Source: three-view drawing plus pictorial views. Frame: mm from the lowest corner of the part. A direction names the side the tool comes from. Coordinates: 2 decimals unless noted, no trailing zeros. Order: outer loops, then holes, each group sorted by start corner. A loop starts at its lowest first (then second) coordinate and runs counter-clockwise, first axis right, second up. Notation, with made-up numbers: (54.5, 83) -> (102.5, 83) arc R12 ccw to (102.5, 103) -> close; hole circle Ø6 at (25, 60.25). An arc over 180 degrees is marked (long way). Use one line per item in the form item = value. Start each with the question number.
1) Ray query, line 1 along Z through (x, y) = (132.5, 16.5); line 2 along X through (y, z) = (7.5, 15); line 3 along Y through (x, z) = (85.5, 62.5). Return the intervals inside material, ascending.
2) Section query A-A on y = 21. Output: boundary loops of the cut face in (x, z).
3) Section query B-B on z = 40. Output: boundary loops of the cut face in (x, y), then the cut area to 3 significant figures.
4) Draft query along X for the marked faces 1, 2, 3 and 4. Return one class per face: pulls with the +X half, pulls with the -X half, needs draft (parallel to the pull), parting line crosses it, or undercut.
5) Pin query (flat end, axial travel): pin 1 (8 mm diameter, centred on x = 114, z = 23, fed in from +Y). Return the tip coordinate at first contact, or that it passes through.
6) Section query C-C on x = 145.5. Output: boundary loops of the cut face in (y, z).
7) Access query for the marked faces 5 and 6. Directions: +Z, -Z, +X, -X, +Y, -Y. A direction counts if a zero-diameter tool reaches every point of the face in a straight line with its end or side. Return the directions, or none.
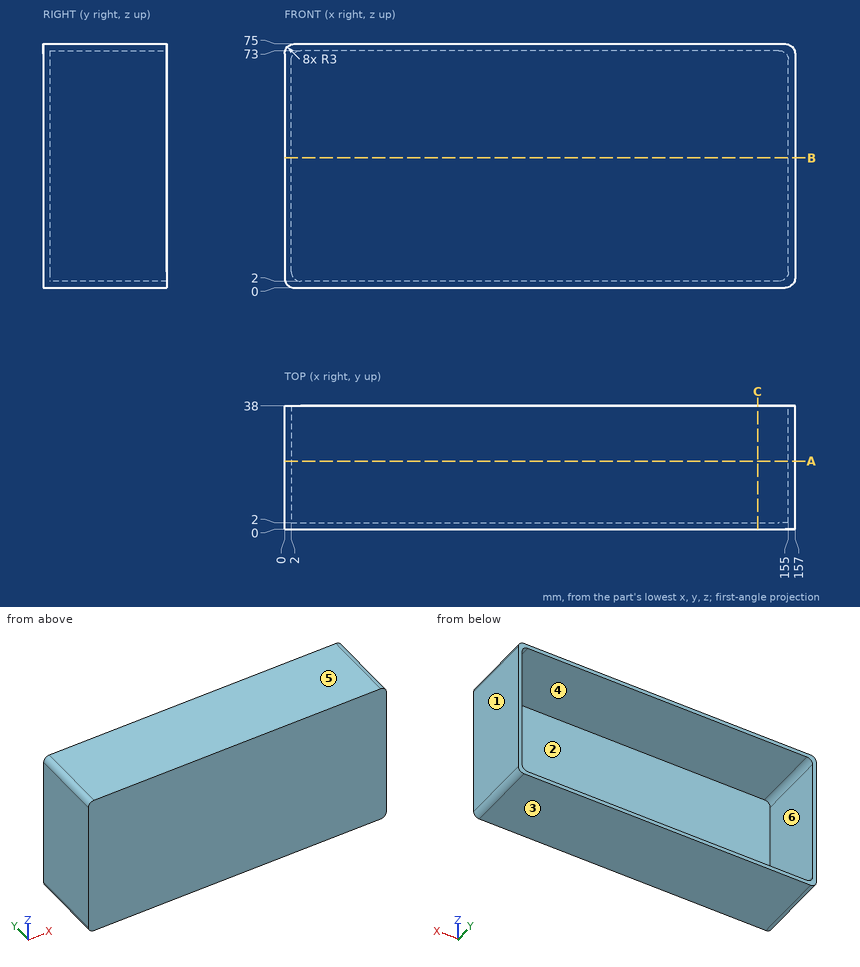
Answers below:
q1.line_1 = 0 to 2, 73 to 75
q1.line_2 = 0 to 2, 155 to 157
q1.line_3 = 0 to 2
q2.outline = (0, 3) arc R3 ccw to (3, 0) -> (154, 0) arc R3 ccw to (157, 3) -> (157, 72) arc R3 ccw to (154, 75) -> (3, 75) arc R3 ccw to (0, 72) -> close; hole (2, 5) arc R3 ccw to (5, 2) -> (152, 2) arc R3 ccw to (155, 5) -> (155, 70) arc R3 ccw to (152, 73) -> (5, 73) arc R3 ccw to (2, 70) -> close
q3.outline = (0, 0) -> (157, 0) -> (157, 38) -> (155, 38) -> (155, 2) -> (2, 2) -> (2, 38) -> (0, 38) -> close
q3.area = 458 mm^2
q4.face_1 = pulls with the +X half
q4.face_2 = undercut
q4.face_3 = needs draft
q4.face_4 = undercut
q5.pin_1 = 2
q6.outline = (0, 0) -> (38, 0) -> (38, 2) -> (2, 2) -> (2, 73) -> (38, 73) -> (38, 75) -> (0, 75) -> close
q7.face_5 = +Z, +X, -X, +Y, -Y
q7.face_6 = +Y
